Work out the finished part from the listing and answer in its coordinate system (mm). Coordinates: 2 decimals unless noted, no trailing zeros. Loops run counter-clockwise (first coordinate to the right, second up) from the corner with the lowest first, then second, coordinate; pieces in that order, holes last. Notation, with made-up numbers: (33, 36) - (69, 36) arc R29 cw to (69, 61) - close; hole circle Ø6 at (84.5, 30). An arc over 180 degrees is marked (long way). Write each question's results on one line, items separated by ' | '. Start each with the question number.
1. A cutting plane is placed at A-A on x = 62. Determine the outline of the cut face in (y, z).
2. A cutting plane is placed at B-B on y = 170. Determine the outline of the cut face in (x, z).
3. A cutting plane is placed at C-C on z = 1.3. State how many separate pieces and enclosed holes the cut face has, then the cut area to 3 significant figures.
4. Find the intervals of material crossed by line 1 along X through (y, z) = (213, 2.6); line 2 along Y through (x, z) = (226.5, 2.25); line 3 along Y through (x, z) = (139, 2.05), in increasing order. Write a range as [from, to].
Autodesk Inventor part; units mm, degrees
ref_plane "YZ Plane" through (0, 0, 0) normal (1, 0, 0) x (0, 1, 0)
ref_plane "XZ Plane" through (0, 0, 0) normal (0, 1, 0) x (-1, 0, 0)
ref_plane "XY Plane" through (0, 0, 0) normal (0, 0, 1) x (1, 0, 0)
sketch "Sketch1" plane through (0, 0, 0) normal (0, 0, 1) x (1, 0, 0)
  line L0 (0, 0) -> (236.5, 0)
  line L1 (236.5, 0) -> (236.5, 296)
  line L2 (236.5, 296) -> (0, 296)
  line L3 (0, 296) -> (0, 0)
  dimension "d0" = 236.5
  dimension "d1" = 296
extrude "Extrusion1" add sketch "Sketch1" along normal blind 3
sketch "Sketch2" plane through (0, 0, 3) normal (0, 0, 1) x (1, 0, 0)
  line L0 (0, 0) -> (236.5, 0)
  line L1 (236.5, 0) -> (236.5, 296)
  line L2 (236.5, 296) -> (0, 296)
  line L3 (0, 296) -> (0, 0)
  line L4 (207.5752, 278) -> (27.5752, 278)
  line L5 (27.5752, 278) -> (53.2221, 223)
  line L6 (53.2221, 223) -> (179.8118, 223)
  line L7 (179.8118, 223) -> (207.5752, 278)
  line L8 (216.5, 264.6127) -> (190.1661, 212.4446)
  line L9 (190.1661, 212.4446) -> (216.5, 186.1108)
  line L10 (218.5, 164.3118) -> (179.8118, 203)
  line L11 (216.5, 264.6127) -> (216.5, 186.1108)
  line L12 (179.8118, 203) -> (53.2221, 203)
  line L13 (53.2221, 203) -> (22.7929, 157.529)
  line L14 (18, 265.4073) -> (42.6969, 212.4446)
  line L15 (42.6969, 212.4446) -> (18, 175.5396)
  line L16 (18, 175.5396) -> (18, 265.4073)
  line L17 (22.7929, 138.471) -> (53.2221, 93)
  line L18 (53.2221, 93) -> (179.8118, 93)
  line L19 (179.8118, 93) -> (218.5, 131.6882)
  line L20 (218.5, 131.6882) -> (218.5, 164.3118)
  line L21 (216.5, 109.8892) -> (190.1661, 83.5554)
  line L22 (190.1661, 83.5554) -> (216.5, 31.3873)
  line L23 (216.5, 31.3873) -> (216.5, 109.8892)
  line L24 (18, 120.4604) -> (42.6969, 83.5554)
  line L25 (42.6969, 83.5554) -> (18, 30.5927)
  line L26 (18, 30.5927) -> (18, 120.4604)
  line L27 (27.5752, 18) -> (207.5752, 18)
  line L28 (207.5752, 18) -> (179.8118, 73)
  line L29 (179.8118, 73) -> (53.2221, 73)
  line L30 (53.2221, 73) -> (27.5752, 18)
  line L31 (22.7929, 138.471) -> (22.7929, 157.529)
  dimension "d19" = 65
  dimension "d29" = 110
  dimension "d31" = 20
  dimension "d32" = 18
  dimension "d33" = 18
  dimension "d34" = 20
  dimension "d35" = 18
  dimension "d40" = 14
  dimension "d41" = 14
  dimension "d52" = 180
  dimension "d55" = 135
  dimension "d59" = 20
  dimension "d60" = 14
  dimension "d61" = 14
  dimension "d62" = 14
  dimension "d63" = 14
  dimension "d64" = 18
extrude "Extrusion2" cut sketch "Sketch2" against normal up to next contours L7 L6 L5 L4 | L11 L9 L8 | L20 L19 L18 L17 L31 L13 L12 L10 | L14 L15 L16 | L23 L22 L21 | L24 L25 L26 | L30 L29 L28 L27
sketch "Sketch3" plane through (0, 0, 3) normal (0, 0, 1) x (1, 0, 0)
  line L0 (0, 0) -> (236.5, 0)
  line L1 (236.5, 0) -> (236.5, 296)
  line L2 (236.5, 296) -> (0, 296)
  line L3 (0, 296) -> (0, 0)
  circle A0 centre (222.5, 282) radius 2.25
  circle A1 centre (14, 148) radius 2.25
  circle A2 centre (222.5, 14) radius 2.25
  dimension "d44" = 4.5
  dimension "d45" = 14
  dimension "d46" = 14
  dimension "d47" = 14
  dimension "d56" = 148
  dimension "d57" = 14
extrude "Extrusion3" cut sketch "Sketch3" against normal up to next contours A0 | A1 | A2
fillet "Fillet1" radius 4.7625 28 edges at (27.5752, 18, 1.5) (207.5752, 18, 1.5) (179.8118, 73, 1.5) (53.2221, 73, 1.5) (18, 30.5927, 1.5) (42.6969, 83.5554, 1.5) (18, 120.4604, 1.5) (42.6969, 212.4446, 1.5) (18, 175.5396, 1.5) (18, 265.4073, 1.5) (27.5752, 278, 1.5) (53.2221, 223, 1.5) (179.8118, 223, 1.5) (207.5752, 278, 1.5) (190.1661, 83.5554, 1.5) (216.5, 31.3873, 1.5) (216.5, 109.8892, 1.5) (216.5, 186.1108, 1.5) (190.1661, 212.4446, 1.5) (216.5, 264.6127, 1.5) (218.5, 131.6882, 1.5) (218.5, 164.3118, 1.5) (179.8118, 93, 1.5) (179.8118, 203, 1.5) (53.2221, 203, 1.5) (22.7929, 157.529, 1.5) (22.7929, 138.471, 1.5) (53.2221, 93, 1.5)
fillet "Fillet2" radius 5 4 edges at (236.5, 0, 1.5) (0, 0, 1.5) (0, 296, 1.5) (236.5, 296, 1.5)
sketch "Sketch4" plane through (0, 0, 0) normal (0, 0, -1) x (-1, 0, 0)
  line L0 (-177.8391, 203) -> (-55.7656, 203)
  line L1 (-55.7656, 93) -> (-177.8391, 93)
  line L2 (-236.5, 5) -> (-236.5, 291)
  line L3 (0, 291) -> (0, 5)
  point P0 (0, 0)
  point P1 (-10, 213)
  point P2 (-226.5, 213)
  point P3 (-10, 83)
  point P4 (-226.5, 83)
  dimension "d65" = 10
  dimension "d66" = 10
  dimension "d67" = 10
  dimension "d68" = 10
hole "Hole1" at (10, 213, 0) at (226.5, 213, 0) at (10, 83, 0) at (226.5, 83, 0) direction (0, 0, 1) diameter 4 end through all countersink diameter 8 countersink angle 90
properties part number "ZBedPlate" material "Steel, Alloy"
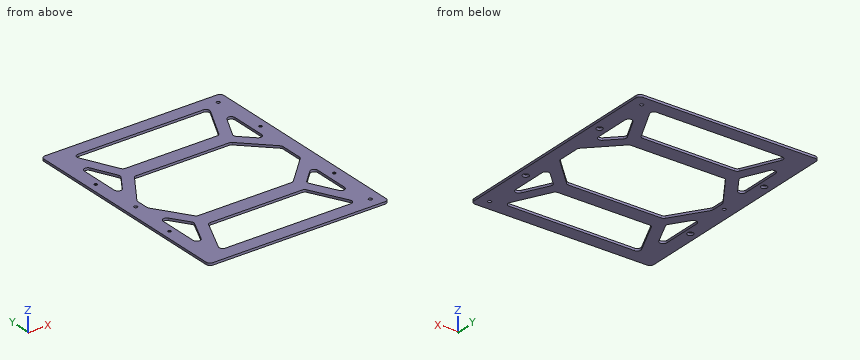
Values:
1) outline: (0, 0) - (18, 0) - (18, 3) - (0, 3) - close; (73, 0) - (93, 0) - (93, 3) - (73, 3) - close; (203, 0) - (223, 0) - (223, 3) - (203, 3) - close; (278, 0) - (296, 0) - (296, 3) - (278, 3) - close
2) outline: (0, 0) - (31.14, 0) - (31.14, 3) - (0, 3) - close; (212.81, 0) - (236.5, 0) - (236.5, 3) - (212.81, 3) - close
3) separate pieces: 1 | enclosed holes: 14 | area: 30,500 mm^2
4) line 1: [0, 8], [12, 18], [42.01, 191.22], [216.5, 224.5], [228.5, 236.5] | line 2: [0, 81], [85, 211], [215, 296] | line 3: [0, 18], [73, 93], [203, 223], [278, 296]
